from build123d import *

# Parameters (mm, degrees)
F2_SIZE = 5
F3_SIZE = 0.5
F4_R    = 1


with BuildPart() as f1:
    # F0 (on Front) → F1 (revolve)
    with BuildSketch(Plane.XZ):
        Polygon((15, 2), (0, 2), (0, 0), (30, 0), (30, 7), (15, 7), align=None)
    revolve(axis=Axis((0, 0, 16.768291272), (0, 0, -1)))

    # F2
    f2_edges = [f1.edges().sort_by_distance(p)[0] for p in [
        (-30, 0, 7),
    ]]
    chamfer(f2_edges, length=F2_SIZE)

    # F3
    f3_edges = [f1.edges().sort_by_distance(p)[0] for p in [
        (-15, 0, 7),
    ]]
    chamfer(f3_edges, length=F3_SIZE)

    # F4
    f4_edges = [f1.edges().sort_by_distance(p)[0] for p in [
        (-25, 0, 7),
        (-30, 0, 2),
    ]]
    fillet(f4_edges, radius=F4_R)


solid = f1.part
Geometry: final body of the model. Coordinates: model frame, mm. A direction names the side the tool comes from. Coordinates: 2 decimals unless noted, no trailing zeros. Loops run counter-clockwise (first coordinate to the right, second up) from the corner with the lowest first, then second, coordinate; pieces in that order, holes last. Notation, with made-up numbers: (-24, -13) - (35, -13) arc R33 ccw to (35, 23) - close; hole circle Ø8 at (-28.75, 21.25). An arc over 180 degrees is marked (long way). One line per question, with ' | ' between items. Start each with the question number.
(1) Draft query along X for faces 3 (the conical face through (24, 10, 6)), 4 (the cylindrical face through (-14.985, -0.66, 4.219)), 5 (the flat face through (0, 0, 0)). Return one class per face: +X half, -X half, draft (parallel to the pull), parting line (faces both ways), or undercut.
(2) Cut plane A-A on z = 5. Output: boundary loops of the cut face in (x, y), and give its area (3 significant figures).
(3) First-contact query: pin 1 (4 mm diameter, centred on x = 18.5, z = 5.5, fed in from +Y). Flat tip, straight axial feed; report the tip coordinate or a pass-through.
(4) Ray query, L1, parallel to X at y = 13.5, z = 5.25; L2, parallel to X at y = 0, z = 3.95; L3, parallel to Y at x = 23, z = 4.25. Return the intervals inside material, ascending. Write a range as from..to.
(5) Reachability of faces 1 (the flat face through (0, 0, 2)), 2 (the flat face through (16, 0, 7)) from +Z, -Z, +X, -X, +Y, -Y: full face, straight path, thin tool, end or side. Return the list, or none.
Here are the results:
1) face 3: parting line | face 4: undercut | face 5: draft
2) outline: circle Ø54 at (0, 0); hole circle Ø30 at (0, 0) | area: 1,580 mm²
3) pin 1: y = 22.16
4) L1: -23.09..-6.54, 6.54..23.09 | L2: -28.05..-15, 15..28.05 | L3: -15.53..15.53
5) face 1: +Z | face 2: +Z, +X, -X, +Y, -Y
